```python
from build123d import *

# Parameters (mm, degrees)
F0_W         = 15
F0_H         = 40
F1_DEPTH     = 3
F2_R         = 0.5
F3_T1_DEPTH  = 3
F3_T4_ANGLE  = 90
F3_T6_ANGLE  = 90
F3_T8_ANGLE  = 90
F3_T10_ANGLE = 90
F3_T12_ANGLE = 90
F3_T14_ANGLE = 90
F3_T16_ANGLE = 90
F3_T18_ANGLE = 90
F4_R         = 4.1479676184
F5_DEPTH     = 25


# Not quite as in the source:
# - a fillet or chamfer that OpenCascade refuses, or shapes differently, is made with other operations: its cross-section is extruded or revolved along the edge and cut away or added


with BuildPart() as f1:
    # F0 (on Top) → F1 (new body)
    with BuildSketch(Plane.XY):
        with Locations((7.5, -20)):
            Rectangle(F0_W, F0_H)
    extrude(amount=F1_DEPTH)

    # F2
    f2_edges = [f1.edges().sort_by_distance(p)[0] for p in [
        (15, -20, 3),
        (7.5, 0, 3),
        (0, -20, 3),
        (7.5, -40, 3),
        (15, -20, 0),
        (7.5, 0, 0),
        (0, -20, 0),
        (7.5, -40, 0),
    ]]
    fillet(f2_edges, radius=F2_R)

    # F3: fillet of radius 7 on 4 edges, made by hand

    # F3_s2 → F3_t1 (cut)
    with BuildSketch(Plane.XY):
        with BuildLine():
            ThreePointArc((15, -7), (12.9497474683, -2.0502525317), (8, 0))
            Line((8, 0), (15, 0))
            Line((15, 0), (15, -7))
        make_face()
        with BuildLine():
            ThreePointArc((7, 0), (2.0502525317, -2.0502525317), (0, -7))
            Line((0, -7), (0, 0))
            Line((0, 0), (7, 0))
        make_face()
        with BuildLine():
            ThreePointArc((15, -33), (12.9497474683, -37.9497474683), (8, -40))
            Line((8, -40), (15, -40))
            Line((15, -40), (15, -33))
        make_face()
        with BuildLine():
            ThreePointArc((7, -40), (2.0502525317, -37.9497474683), (0, -33))
            Line((0, -33), (0, -40))
            Line((0, -40), (7, -40))
        make_face()
    extrude(amount=F3_T1_DEPTH, mode=Mode.SUBTRACT)

    # F3_s3 → F3_t4 (revolve, cut)
    with BuildSketch(Plane.YZ.offset(7)):
        with BuildLine():
            ThreePointArc((-39.5, 0), (-39.8535533906, 0.1464466094), (-40, 0.5))
            Line((-40, 0.5), (-40, 0))
            Line((-40, 0), (-39.5, 0))
        make_face()
    revolve(axis=Axis((7, -33, 0), (0, 0, -1)), revolution_arc=F3_T4_ANGLE, mode=Mode.SUBTRACT)

    # F3_s5 → F3_t6 (revolve, cut)
    with BuildSketch(Plane.XZ.offset(33)):
        with BuildLine():
            ThreePointArc((0.5, 3), (0.1464466094, 2.8535533906), (0, 2.5))
            Line((0, 2.5), (0, 3))
            Line((0, 3), (0.5, 3))
        make_face()
    revolve(axis=Axis((7, -33, 3), (0, 0, 1)), revolution_arc=F3_T6_ANGLE, mode=Mode.SUBTRACT)

    # F3_s7 → F3_t8 (revolve, cut)
    with BuildSketch(Plane.XZ.offset(33)):
        with BuildLine():
            ThreePointArc((14.5, 0), (14.8535533906, 0.1464466094), (15, 0.5))
            Line((15, 0.5), (15, 0))
            Line((15, 0), (14.5, 0))
        make_face()
    revolve(axis=Axis((8, -33, 0), (0, 0, -1)), revolution_arc=F3_T8_ANGLE, mode=Mode.SUBTRACT)

    # F3_s9 → F3_t10 (revolve, cut)
    with BuildSketch(Plane.YZ.offset(8)):
        with BuildLine():
            ThreePointArc((-39.5, 3), (-39.8535533906, 2.8535533906), (-40, 2.5))
            Line((-40, 2.5), (-40, 3))
            Line((-40, 3), (-39.5, 3))
        make_face()
    revolve(axis=Axis((8, -33, 3), (0, 0, 1)), revolution_arc=F3_T10_ANGLE, mode=Mode.SUBTRACT)

    # F3_s11 → F3_t12 (revolve, cut)
    with BuildSketch(Plane.XZ.offset(7)):
        with BuildLine():
            ThreePointArc((0.5, 0), (0.1464466094, 0.1464466094), (0, 0.5))
            Line((0, 0.5), (0, 0))
            Line((0, 0), (0.5, 0))
        make_face()
    revolve(axis=Axis((7, -7, 0), (0, 0, -1)), revolution_arc=F3_T12_ANGLE, mode=Mode.SUBTRACT)

    # F3_s13 → F3_t14 (revolve, cut)
    with BuildSketch(Plane.YZ.offset(7)):
        with BuildLine():
            ThreePointArc((-0.5, 3), (-0.1464466094, 2.8535533906), (0, 2.5))
            Line((0, 2.5), (0, 3))
            Line((0, 3), (-0.5, 3))
        make_face()
    revolve(axis=Axis((7, -7, 3), (0, 0, 1)), revolution_arc=F3_T14_ANGLE, mode=Mode.SUBTRACT)

    # F3_s15 → F3_t16 (revolve, cut)
    with BuildSketch(Plane.YZ.offset(8)):
        with BuildLine():
            ThreePointArc((-0.5, 0), (-0.1464466094, 0.1464466094), (0, 0.5))
            Line((0, 0.5), (0, 0))
            Line((0, 0), (-0.5, 0))
        make_face()
    revolve(axis=Axis((8, -7, 0), (0, 0, -1)), revolution_arc=F3_T16_ANGLE, mode=Mode.SUBTRACT)

    # F3_s17 → F3_t18 (revolve, cut)
    with BuildSketch(Plane.XZ.offset(7)):
        with BuildLine():
            ThreePointArc((14.5, 3), (14.8535533906, 2.8535533906), (15, 2.5))
            Line((15, 2.5), (15, 3))
            Line((15, 3), (14.5, 3))
        make_face()
    revolve(axis=Axis((8, -7, 3), (0, 0, 1)), revolution_arc=F3_T18_ANGLE, mode=Mode.SUBTRACT)

    # F4 (on face) → F5 (cut)
    with BuildSketch(Plane.XY.offset(3)):
        with Locations((6.9764298387, -7.8903073445)):
            Circle(F4_R)
    extrude(amount=-F5_DEPTH, mode=Mode.SUBTRACT)


solid = f1.part
```
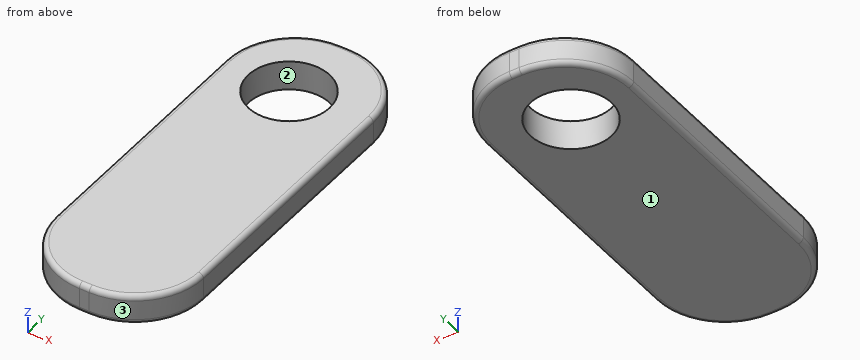
Verification items for the finished model (mm, model axes). Face numbers are marked on the shaded views. Coordinates: 2 decimals unless noted, no trailing zeros. Loops run counter-clockwise (first coordinate to the right, second up) from the corner with the lowest first, then second, coordinate; pieces in that order, holes last. Notation, with made-up numbers: (10, -2.75) -> (33, -2.75) arc R26 cw to (33, 12.25) -> close; hole circle Ø1 at (36, -22). An arc over 180 degrees is marked (long way). Answer in a Markdown table with one row per item. Add a question column.
1. Depth check by flat-ended pin: P1, Ø5, axis at x = 6.98, y = -7.89, coming from the +Z side; P2, Ø1.5, axis at y = -5, z = 1.5, coming from the -X side. Enter the tip coordinate at first touch or a pass-through.
2. Section check A-A, the plane z = 1.25. Enter the section's corners in (x, y).
3. Material ranges on probe 1 along Y at (x, z) = (4.75, 0.7); probe 2 along X at (y, z) = (-14, 0.45); probe 3 along Y at (x, z) = (6, 0.35), recorded low to high. Write a range as [from, to].
4. Draft check along Y on the marked faces 1, 2 and 3. Enter one of: +Y half, -Y half, draft (parallel to the pull), parting line (faces both ways), or undercut.
Derived:
| question | item | result |
|---|---|---|
| 1 | P1 | passes through |
| 1 | P2 | stops at x = 0.11 |
| 2 | outline | (0, -33) arc R7 ccw to (7, -40) -> (8, -40) arc R7 ccw to (15, -33) -> (15, -7) arc R7 ccw to (8, 0) -> (7, 0) arc R7 ccw to (0, -7) -> close; hole circle Ø8.3 at (6.98, -7.89) |
| 3 | probe 1 | y = [-39.63, -11.39], [-4.39, -0.37] |
| 3 | probe 2 | x = [0, 15] |
| 3 | probe 3 | y = [-39.9, -11.92], [-3.86, -0.1] |
| 4 | face 1 | draft |
| 4 | face 2 | undercut |
| 4 | face 3 | -Y half |
